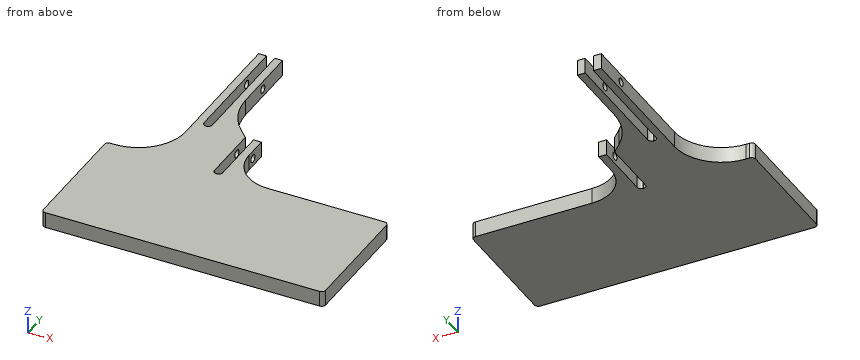
Autodesk Inventor part; units mm, degrees
ref_plane "YZ Plane" through (0, 0, 0) normal (1, 0, 0) x (0, 1, 0)
ref_plane "XZ Plane" through (0, 0, 0) normal (0, 1, 0) x (-1, 0, 0)
ref_plane "XY Plane" through (0, 0, 0) normal (0, 0, 1) x (1, 0, 0)
sketch "Sketch1" plane through (0, 0, 0) normal (0, 0, 1) x (1, 0, 0)
  line L0 (0, 0) -> (114.3, 0)
  line L1 (0, 0) -> (0, -50.8)
  line L2 (0, -50.8) -> (114.3, -50.8)
  line L3 (114.3, -50.8) -> (114.3, 0)
  dimension "d1" = 114.3
  dimension "d2" = 50.8
  dimension "d3" = 114.3
extrude "Extrusion1" add sketch "Sketch1" along normal blind 3.175
sketch "Sketch2" plane through (0, 0, 0) normal (0, 1, 0) x (1, 0, 0)
  line L0 (114.3, -3.175) -> (0, -3.175)
  line L1 (25.3873, -1.5875) -> (25.3873, 0)
  line L2 (25.3873, -3.175) -> (25.3873, -1.5875)
  line L3 (28.7401, -1.5875) -> (28.7401, -3.175)
  line L4 (28.7401, -1.5875) -> (28.7401, 0)
  line L5 (25.3873, -3.175) -> (22.2123, -3.175)
  line L6 (22.2123, -3.175) -> (22.2123, 3.175)
  line L7 (28.7401, -3.175) -> (31.9151, -3.175)
  line L8 (31.9151, -3.175) -> (31.9151, 3.175)
  line L9 (25.3873, 0) -> (25.3873, 3.175)
  line L10 (25.3873, 3.175) -> (22.2123, 3.175)
  line L11 (31.9151, 3.175) -> (28.7401, 3.175)
  line L12 (28.7401, 3.175) -> (28.7401, 0)
  point P0 (27.0637, -1.5875)
  dimension "d7" = 1.6764
  dimension "d8" = 1.6764
  dimension "d9" = 3.175
  dimension "d10" = 6.35
  dimension "d11" = 3.175
sketch "Sketch3" plane through (0, 0, 0) normal (0, 0, -1) x (-1, 0, 0)
  line L0 (-114.3, 0) -> (0, 0)
  line L1 (0, -50.8) -> (-114.3, -50.8)
  line L2 (0, 0) -> (-114.3, 0)
  line L3 (-114.3, 0) -> (-114.3, -50.8)
  line L4 (-114.3, -50.8) -> (0, -50.8)
  line L5 (0, -50.8) -> (0, 0)
extrude "Extrusion2" add sketch "Sketch3" along normal blind 3.175
extrude "Extrusion3" add sketch "Sketch2" along normal blind 76.2 contours L0 L3 L4 L12 L11 L8
extrude "Extrusion4" add sketch "Sketch2" along normal blind 76.2 contours L0 L6 L10 L9 L1 L2
sketch "Sketch4" plane through (31.9151, 0, 3.175) normal (1, 0, 0) x (0, 0, -1)
  line L0 (3.175, 0) -> (3.175, 19.05)
  circle A0 centre (3.175, 19.05) radius 1.5875
  dimension "d18" = 19.05
  dimension "d19" = 3.175
extrude "Extrusion5" cut sketch "Sketch4" along normal mid plane 50.8
sketch "Sketch5" plane through (31.9151, 0, 3.175) normal (1, 0, 0) x (0, 0, -1)
  circle A0 centre (3.175, 19.05) radius 1.5875
  line L0 (3.175, 19.05) -> (3.175, 60.706)
  circle A1 centre (3.175, 60.706) radius 1.5875
  point P0 (3.175, 0)
  dimension "d22" = 41.656
  dimension "d23" = 3.175
extrude "Extrusion6" cut sketch "Sketch5" against normal blind 50.8 contours A1
sketch "Sketch6" plane through (25.3873, 0, 3.175) normal (1, 0, 0) x (0, 0, -1)
  point P0 (3.175, 0)
sketch "Sketch7" plane through (0, 0, 3.175) normal (0, 0, 1) x (1, 0, 0)
  point P0 (0, 0)
sketch "Sketch8" plane through (0, 0, 3.175) normal (0, 0, 1) x (1, 0, 0)
  line L0 (38.0873, 0) -> (41.2623, 0)
  line L1 (41.2623, 0) -> (41.2623, 22.5425)
  line L2 (38.0873, 0) -> (38.0873, 22.5425)
  line L3 (38.0873, 22.5425) -> (41.2623, 22.5425)
  line L4 (38.0873, 22.5425) -> (31.9151, 22.5425)
  line L5 (31.9151, 0) -> (31.9151, 76.2)
  line L6 (41.2623, 22.5425) -> (41.2623, 25.7175)
  line L7 (41.2623, 25.7175) -> (31.9151, 25.7175)
  point P0 (0, 0)
  dimension "d30" = 3.175
  dimension "d34" = 3.175
sketch "Sketch9" plane through (0, 0, 3.175) normal (0, 0, 1) x (1, 0, 0)
  line L0 (41.2623, 25.7175) -> (41.2623, 0)
  line L1 (31.9151, 0) -> (114.3, 0)
  line L2 (44.6151, 0) -> (44.6151, 25.6324)
  line L3 (44.6151, 25.6324) -> (47.7901, 25.6324)
  line L4 (47.7901, 0) -> (47.7901, 25.6324)
  line L5 (44.6151, 0) -> (47.7901, 0)
  point P0 (0, 0)
  dimension "d35" = 3.3528
  dimension "d36" = 3.175
sketch "Sketch12" plane through (0, 0, 3.175) normal (0, 0, 1) x (1, 0, 0)
  line L0 (44.6151, 0) -> (44.6151, 25.6324)
  line L1 (44.6151, 0) -> (46.3169, 0)
  line L2 (46.3169, 0) -> (49.4919, 0)
  line L3 (25.3873, 0) -> (114.3, 0)
  line L4 (49.4919, 0) -> (49.4919, 25.6324)
  line L5 (49.4919, 25.6324) -> (46.3169, 25.6324)
  line L6 (46.3169, 25.6324) -> (46.3169, 0)
  point P0 (0, 0)
  point P1 (47.7901, 0)
  point P2 (41.2623, 0)
  dimension "d44" = 1.7018
  dimension "d45" = 3.175
extrude "Extrusion11" add sketch "Sketch12" against normal blind 6.35
sketch "Sketch13" plane through (0, 0, 3.175) normal (0, 0, 1) x (1, 0, 0)
  line L0 (38.0873, 22.5425) -> (38.0873, 0)
  line L1 (38.0873, 0) -> (39.7891, 0)
  line L2 (39.7891, 0) -> (42.9641, 0)
  line L3 (46.3169, 0) -> (31.9151, 0)
  line L4 (39.7891, 0) -> (39.7891, 25.7175)
  line L5 (41.2623, 25.7175) -> (31.9151, 25.7175)
  line L6 (42.9641, 0) -> (42.9641, 25.7175)
  line L7 (42.9641, 25.7175) -> (39.7891, 25.7175)
  point P0 (0, 0)
  point P1 (41.2623, 0)
  dimension "d48" = 1.7018
  dimension "d49" = 3.175
extrude "Extrusion12" add sketch "Sketch13" against normal blind 6.35
sketch "Sketch14" plane through (0, 0, 3.175) normal (0, 0, 1) x (1, 0, 0)
  line L0 (39.7891, 25.7175) -> (42.9641, 25.7175)
  line L1 (39.7891, 25.7175) -> (39.7891, 22.5425)
  line L2 (39.7891, 25.7175) -> (39.7891, 0)
  line L3 (39.7891, 22.5425) -> (31.9151, 22.5425)
  line L4 (39.7891, 25.7175) -> (50.9246, 25.7175) construction
  line L5 (42.9641, 25.7175) -> (56.7757, 25.7175) construction
  line L6 (31.9151, 0) -> (31.9151, 76.2)
  line L7 (31.9151, 36.7665) -> (42.9641, 25.7175)
  line L8 (31.9151, 36.7665) -> (31.9151, 22.5425)
  line L9 (42.9641, 25.7175) -> (39.7891, 25.7175)
  line L10 (39.7891, 25.7175) -> (42.9641, 25.7175)
  point P0 (0, 0)
  dimension "d52" = 3.175
extrude "Extrusion13" add sketch "Sketch14" against normal blind 6.35
sketch "Sketch15" plane through (22.2123, 0, -3.175) normal (-1, 0, 0) x (0, 0, 1)
  circle A0 centre (3.175, 19.05) radius 1.5875
  circle A1 centre (3.175, 19.05) radius 1.5875
  point P0 (3.175, 0)
extrude "Extrusion14" cut sketch "Sketch15" against normal blind 50.8
sketch "Sketch16" plane through (0, 0, 3.175) normal (0, 0, 1) x (1, 0, 0)
  line L0 (31.9151, 36.7665) -> (42.9641, 25.7175)
  line L1 (42.9641, 25.7175) -> (22.2123, 25.7175)
  line L2 (22.2123, 0) -> (22.2123, 76.2)
  line L3 (42.9641, 25.7175) -> (42.9641, 0)
  line L4 (42.9641, 0) -> (22.2123, 0)
  line L5 (22.2123, 0) -> (22.2123, 25.7175)
  line L6 (42.9641, 25.7175) -> (42.9641, 0)
  point P0 (0, 0)
extrude "Extrusion15" add sketch "Sketch16" against normal blind 6.35
sketch "Sketch17" plane through (49.4919, 0, 3.175) normal (1, 0, 0) x (0, 0, -1)
  circle A0 centre (3.175, 19.05) radius 1.5875
  circle A1 centre (3.175, 19.05) radius 1.5875
  point P0 (3.175, 0)
extrude "Extrusion16" cut sketch "Sketch17" against normal blind 12.7
fillet "Fillet1" radius 1.5875 2 edges at (42.9641, 0, 0) (46.3169, 0, 0)
fillet "Fillet3" radius 25.4 1 edges at (31.9151, 36.7665, 0)
fillet "Fillet4" radius 1.5875 6 edges at (0, 0, 0) (0, -50.8, 0) (114.3, -50.8, 0) (114.3, 0, 0) (25.3873, 25.7175, 0) (28.7401, 25.7175, 0)
fillet "Fillet5" radius 15.875 1 edges at (49.4919, 0, 0)
fillet "Fillet6" radius 19.05 1 edges at (22.2123, 0, 0)
properties part number "2BarClawPaddle" material "Aluminum 6061"
The model under review builds one solid part; all positions refer to its coordinate system, in mm. Round coordinates to 2 decimals unless told otherwise and drop trailing zeros. Loops run counter-clockwise (first coordinate to the right, second up) from the corner with the lowest first, then second, coordinate; pieces in that order, holes last.
1) Wall thickness on line 1 along Z through (x, y) = (48.45, 19.05) (1 decimal); line 2 along X through (y, z) = (51, -1.75); line 3 along Y through (x, z) = (65, -1.5): over which ranges is each line inside the solid? List them lowest first.
Values follow:
line 1: z = -3.2 to -1.6, 1.6 to 3.2
line 2: x = 22.21 to 25.39, 28.74 to 31.92
line 3: y = -50.8 to 0
2) Consider section A-A on y = 67. State the section outline as (x, z) points (3 decimals), then the cut area to 3 significant figures.
Values follow:
outline: (22.212, -3.175) - (25.387, -3.175) - (25.387, 3.175) - (22.212, 3.175) - close; (28.74, -3.175) - (31.915, -3.175) - (31.915, 3.175) - (28.74, 3.175) - close
area: 40.3 mm2
3) Clearance check with flat-ended pins moving along their axes: P1, Ø3, axis at y = 41, z = -0.5, coming from the -X side; P2, Ø3.5, axis at y = 19.05, z = 0, coming from the -X side; P3, Ø1, axis at y = 18.5, z = 0, coming from the +X side. State where each tip first meets the part, or that it passes through.
Values follow:
P1: stops at x = 22.21
P2: stops at x = 22.13
P3: stops at x = 36.79
4) Consider section D-D on x = 52.5. State the section outline as (y, z) points (3 decimals).
Values follow:
outline: (-50.8, -3.175) - (6.577, -3.175) - (6.577, 3.175) - (-50.8, 3.175) - close
5) Consider section C-C on y = 44.5. State the section outline as (x, z) points (3 decimals).
Values follow:
outline: (22.212, -3.175) - (25.387, -3.175) - (25.387, 3.175) - (22.212, 3.175) - close; (28.74, -3.175) - (32.069, -3.175) - (32.069, 3.175) - (28.74, 3.175) - close
6) Consider section B-B on z = 0. Give the number of separate pieces and of enclosed holes in the cut face, then the cut area to 3 significant figures.
Values follow:
separate pieces: 4
enclosed holes: 0
area: 6,900 mm2
